```python
from build123d import *

# Parameters (mm, degrees)
F0_W     = 815
F0_H     = 1975
F0_W_2   = 610
F0_H_2   = 392.25
F1_DEPTH = 22.5
F2_SIZE2 = 17
F2_SIZE  = 6
F3_SIZE2 = 13
F3_SIZE  = 6
F4_W     = 10
F4_H     = 23
F5_DEPTH = 1975.001


with BuildPart() as f1:
    # F0 (on Front) → F1 (new body, symmetric)
    with BuildSketch(Plane.XZ):
        Rectangle(F0_W, F0_H)
        with Locations((0, -551.375)):
            Rectangle(F0_W_2, F0_H_2, mode=Mode.SUBTRACT)
        with Locations((0, -137.125)):
            Rectangle(F0_W_2, F0_H_2, mode=Mode.SUBTRACT)
        with Locations((0, 277.125)):
            Rectangle(F0_W_2, F0_H_2, mode=Mode.SUBTRACT)
        with Locations((0, 691.375)):
            Rectangle(F0_W_2, F0_H_2, mode=Mode.SUBTRACT)
    extrude(amount=F1_DEPTH, both=True)

    # F2
    f2_edges = [f1.edges().sort_by_distance(p)[0] for p in [
        (305, -22.5, -551.375),
        (0, -22.5, -355.25),
        (305, -22.5, -137.125),
        (0, -22.5, 59),
        (305, -22.5, 277.125),
        (0, -22.5, 473.25),
        (305, -22.5, 691.375),
        (0, -22.5, 887.5),
        (-305, -22.5, 691.375),
        (0, -22.5, 495.25),
        (-305, -22.5, 277.125),
        (0, -22.5, 81),
        (-305, -22.5, -137.125),
        (0, -22.5, -333.25),
        (-305, -22.5, -551.375),
        (0, -22.5, -747.5),
    ]]
    f2_side = f1.faces().sort_by_distance((0, -22.5, 966.13449))[0]
    chamfer(f2_edges, length=F2_SIZE, length2=F2_SIZE2, reference=f2_side)

    # F3
    f3_edges = [f1.edges().sort_by_distance(p)[0] for p in [
        (0, 22.5, -747.5),
        (305, 22.5, -551.375),
        (0, 22.5, -355.25),
        (-305, 22.5, -551.375),
        (-305, 22.5, -137.125),
        (0, 22.5, 59),
        (-305, 22.5, 277.125),
        (0, 22.5, -333.25),
        (305, 22.5, -137.125),
        (0, 22.5, 81),
        (305, 22.5, 277.125),
        (0, 22.5, 473.25),
        (305, 22.5, 691.375),
        (0, 22.5, 887.5),
        (-305, 22.5, 691.375),
        (0, 22.5, 495.25),
    ]]
    f3_side = f1.faces().sort_by_distance((0, 22.5, 966.13449))[0]
    chamfer(f3_edges, length=F3_SIZE, length2=F3_SIZE2, reference=f3_side)

    # F4 (on face) → F5 (cut, through all)
    with BuildSketch(Plane(origin=(0, 0, -987.5), x_dir=(1, 0, 0), z_dir=(0, 0, -1))):
        with Locations((402.5, 11)):
            Rectangle(F4_W, F4_H)
    extrude(amount=-F5_DEPTH, mode=Mode.SUBTRACT)


solid = f1.part
```
Part model, mm, in its own coordinate system. Round coordinates to 2 decimals unless told otherwise and drop trailing zeros. Order: outer loops, then holes, each group sorted by start corner. A loop starts at its lowest first (then second) coordinate and runs counter-clockwise, first axis right, second up. Notation, with made-up numbers: M 46.25,34 L 80.25,34 A29 ccw 80.25,57 Z; hole C 36,62.5 d11. An arc over 180 degrees is marked long. Put each result on its own line as item: value. Start each with the question number.
1. Slice it at A-A on z = 788. List the corners of the cut face in (x, y).
2. Slice it at C-C on x = -228. State how many separate pieces and enclosed holes the cut face has, then the cut area to 4 significant figures.
3. Slice it at B-B on y = -13. List the corners of the cut face in (x, z), then the cut area to 3 significant figures.
4. Drill centre lines: probe 1 along Z at (x, y) = (113, 5.5); probe 2 along Z at (x, y) = (-72.5, -6); probe 3 along X at (y, z) = (2.5, -644). Where is each one in solid material? Low to high. Write a range as [from, to].
5. Drop flat-ended pins along their axis: pin 1 (16.5 mm diameter, centred on y = 0, z = -587.5, fed in from +X); pin 2 (18.5 mm diameter, centred on y = -16, z = -321.5, fed in from +X). Give the stop position or say it passes through.
Findings:
1. outline: M -407.5,-22.5 L -311,-22.5 L -305,-5.5 L -305,9.5 L -311,22.5 L -407.5,22.5 Z; M 305,-5.5 L 311,-22.5 L 397.5,-22.5 L 397.5,0.5 L 407.5,0.5 L 407.5,22.5 L 311,22.5 L 305,9.5 Z
2. separate pieces: 5
2. enclosed holes: 0
2. area: 17,550 mm2
3. outline: M -407.5,-987.5 L 397.5,-987.5 L 397.5,987.5 L -407.5,987.5 Z; hole M -307.65,-750.15 L 307.65,-750.15 L 307.65,-352.6 L -307.65,-352.6 Z; hole M -307.65,-335.9 L 307.65,-335.9 L 307.65,61.65 L -307.65,61.65 Z; hole M -307.65,78.35 L 307.65,78.35 L 307.65,475.9 L -307.65,475.9 Z; hole M -307.65,492.6 L 307.65,492.6 L 307.65,890.15 L -307.65,890.15 Z
3. area: 611,000 mm2
4. probe 1: [-987.5, -747.5], [-355.25, -333.25], [59, 81], [473.25, 495.25], [887.5, 987.5]
4. probe 2: [-987.5, -747.68], [-355.07, -333.43], [59.18, 80.82], [473.43, 495.07], [887.68, 987.5]
4. probe 3: [-407.5, -305], [305, 407.5]
5. pin 1: x = 407.5
5. pin 2: x = 397.5
